```python
from build123d import *

# Parameters (mm, degrees)
F1_DEPTH = 2
F3_DEPTH = 25.4
F4_R     = 20


with BuildPart() as f1:
    # F0 (on Front) → F1 (new body)
    with BuildSketch(Plane.XZ):
        with BuildLine():
            ThreePointArc((177.655664, -174.737987), (195.333333, -167.415657), (202.655664, -149.737987))
            Line((202.655664, -149.737987), (202.655664, 175.262013))
            ThreePointArc((202.655664, 175.262013), (195.333333, 192.939682), (177.655664, 200.262013))
            Line((177.655664, 200.262013), (147.655664, 200.262013))
            Line((147.655664, 200.262013), (117.655664, 185.262013))
            Line((117.655664, 185.262013), (-32.344336, 185.262013))
            Line((-32.344336, 185.262013), (-182.344336, 185.262013))
            Line((-182.344336, 185.262013), (-212.344336, 200.262013))
            Line((-212.344336, 200.262013), (-242.344336, 200.262013))
            ThreePointArc((-242.344336, 200.262013), (-260.022006, 192.939682), (-267.344336, 175.262013))
            Line((-267.344336, 175.262013), (-267.344336, -149.737987))
            ThreePointArc((-267.344336, -149.737987), (-260.022006, -167.415657), (-242.344336, -174.737987))
            Line((-242.344336, -174.737987), (177.655664, -174.737987))
        make_face()
    extrude(amount=F1_DEPTH)

    # F2 (on face) → F3 (cut)
    with BuildSketch(Plane.XZ.offset(2)):
        with BuildLine():
            Line((-116.005836, -51.443487), (51.317164, -51.443487))
            ThreePointArc((51.317164, -51.443487), (52.731377, -50.857701), (53.317164, -49.443487))
            Line((53.317164, -49.443487), (53.317164, 59.967513))
            ThreePointArc((53.317164, 59.967513), (52.731377, 61.381726), (51.317164, 61.967513))
            Line((51.317164, 61.967513), (-116.005836, 61.967513))
            ThreePointArc((-116.005836, 61.967513), (-117.42005, 61.381726), (-118.005836, 59.967513))
            Line((-118.005836, 59.967513), (-118.005836, -49.443487))
            ThreePointArc((-118.005836, -49.443487), (-117.42005, -50.857701), (-116.005836, -51.443487))
        make_face()
    extrude(amount=-F3_DEPTH, mode=Mode.SUBTRACT)

    # F4
    f4_edges = [f1.edges().sort_by_distance(p)[0] for p in [
        (147.655664, -1, 200.262013),
        (117.655664, -1, 185.262013),
        (-212.344336, -1, 200.262013),
        (-182.344336, -1, 185.262013),
    ]]
    fillet(f4_edges, radius=F4_R)


solid = f1.part
```
The listing builds one solid part. Answer for the finished solid, in the listing's coordinates (mm). A direction names the side the tool comes from. Give positions to 0.01 mm unless a question says otherwise; leave off trailing zeros. Order: outer loops, then holes, each group sorted by start corner. A loop starts at its lowest first (then second) coordinate and runs counter-clockwise, first axis right, second up. Notation, with made-up numbers: M -34,37 L 19,37 A14 ccw 19,49 Z; hole C -7,65 d11. An arc over 180 degrees is marked long. Put each result on its own line as item: value. Start each with the question number.
Item 1: The part is cut by section C-C, the plane y = -1.6. Determine the outline of the cut face in (x, z), and give its area (3 significant figures).
Item 2: Find the intervals of material crossed by line 1 along X through (y, z) = (-0.5, 4); line 2 along Z through (x, y) = (-47, -1.2); line 3 along Z through (x, y) = (95, -0.8), in increasing order.
Item 3: The part is cut by section D-D, the plane x = 75. Determine the outline of the cut face in (y, z), and give its area (3 significant figures).
Item 4: The part is cut by section A-A, the plane z = -23.5. Determine the outline of the cut face in (x, y), and give its area (3 significant figures).
Item 5: Which of the six approach directions +Z, -Z, +X, -X, +Y, -Y give full straight-line access (tool end or side, diameter ignored) to faces 1 (the face through (-197.193, -0.986, 192.687)), 2 (the face through (195.138, -0.986, -167.609))?
Item 6: The part is cut by section B-B, the plane x = -103.5. Determine the outline of the cut face in (y, z), and give its area (3 significant figures).
Answer key:
1. outline: M -267.34,-149.74 A25 ccw -242.34,-174.74 L 177.66,-174.74 A25 ccw 202.66,-149.74 L 202.66,175.26 A25 ccw 177.66,200.26 L 152.38,200.26 A20 ccw 143.43,198.15 L 121.88,187.37 A20 cw 112.93,185.26 L -177.62,185.26 A20 cw -186.57,187.37 L -208.12,198.15 A20 ccw -217.07,200.26 L -242.34,200.26 A25 ccw -267.34,175.26 Z; hole M -118.01,-49.44 A2 ccw -116.01,-51.44 L 51.32,-51.44 A2 ccw 53.32,-49.44 L 53.32,59.97 A2 ccw 51.32,61.97 L -116.01,61.97 A2 ccw -118.01,59.97 Z
1. area: 151,000 mm²
2. line 1: x = -267.34 to -118.01, 53.32 to 202.66
2. line 2: z = -174.74 to -51.44, 61.97 to 185.26
2. line 3: z = -174.74 to 185.26
3. outline: M -2,-174.74 L 0,-174.74 L 0,185.26 L -2,185.26 Z
3. area: 720 mm²
4. outline: M -267.34,-2 L -118.01,-2 L -118.01,0 L -267.34,0 Z; M 53.32,-2 L 202.66,-2 L 202.66,0 L 53.32,0 Z
4. area: 597 mm²
5. face 1: +Z, +Y, -Y
5. face 2: -Z, +X, +Y, -Y
6. outline: M -2,-174.74 L 0,-174.74 L 0,-51.44 L -2,-51.44 Z; M -2,61.97 L 0,61.97 L 0,185.26 L -2,185.26 Z
6. area: 493 mm²
